from build123d import *

# Parameters (mm, degrees)
BOSS_EXTRUDE1_DEPTH = 2.54
CUT_EXTRUDE1_DEPTH  = 3.54
CUT_EXTRUDE2_DEPTH  = 3.54


with BuildPart() as part:
    # Sketch1 → Boss-Extrude1 (new body)
    with BuildSketch(Plane(origin=(0, 0, 0), x_dir=(1, 0, 0), z_dir=(0, 1, 0))):
        Polygon((-66.675, 25.4), (-69.215, 25.4), (-69.215, -25.4), (-66.675, -25.4), (-66.675, -27.813), (66.675, -27.813), (66.675, -25.4), (69.215, -25.4), (69.215, 25.4), (66.675, 25.4), (66.675, 27.813), (-66.675, 27.813), align=None)
    extrude(amount=BOSS_EXTRUDE1_DEPTH)

    # Sketch2 → Cut-Extrude1 (cut, through all)
    with BuildSketch(Plane(origin=(0, 2.54, 0), x_dir=(1, 0, 0), z_dir=(0, 1, 0))):
        with BuildLine():
            ThreePointArc((-60.96, 16.51), (-64.212038418, 17.857038418), (-62.865, 14.605))
            Line((-62.865, 14.605), (-62.865, 16.51))
            Line((-62.865, 16.51), (-60.96, 16.51))
        make_face()
        with BuildLine():
            Line((-62.865, 16.51), (-62.865, 14.605))
            ThreePointArc((-62.865, 14.605), (-61.517961582, 15.162961582), (-60.96, 16.51))
            Line((-60.96, 16.51), (-62.865, 16.51))
        make_face()
        with BuildLine():
            ThreePointArc((-19.05, 16.51), (-18.492038418, 15.162961582), (-17.145, 14.605))
            Line((-17.145, 14.605), (-17.145, 16.51))
            Line((-17.145, 16.51), (-19.05, 16.51))
        make_face()
        with BuildLine():
            Line((-17.145, 16.51), (-17.145, 14.605))
            ThreePointArc((-17.145, 14.605), (-15.797961582, 15.162961582), (-15.24, 16.51))
            ThreePointArc((-15.24, 16.51), (-17.145, 18.415), (-19.05, 16.51))
            Line((-19.05, 16.51), (-17.145, 16.51))
        make_face()
        with BuildLine():
            ThreePointArc((-17.145, -14.605), (-18.492038418, -15.162961582), (-19.05, -16.51))
            Line((-19.05, -16.51), (-17.145, -16.51))
            Line((-17.145, -16.51), (-17.145, -14.605))
        make_face()
        with BuildLine():
            Line((-17.145, -16.51), (-19.05, -16.51))
            ThreePointArc((-19.05, -16.51), (-17.145, -18.415), (-15.24, -16.51))
            ThreePointArc((-15.24, -16.51), (-15.797961582, -15.162961582), (-17.145, -14.605))
            Line((-17.145, -14.605), (-17.145, -16.51))
        make_face()
        with BuildLine():
            Line((-62.865, -14.605), (-62.865, -16.51))
            Line((-62.865, -16.51), (-60.96, -16.51))
            ThreePointArc((-60.96, -16.51), (-61.517961582, -15.162961582), (-62.865, -14.605))
        make_face()
        with BuildLine():
            Line((-60.96, -16.51), (-62.865, -16.51))
            Line((-62.865, -16.51), (-62.865, -14.605))
            ThreePointArc((-62.865, -14.605), (-64.212038418, -17.857038418), (-60.96, -16.51))
        make_face()
    extrude(amount=-CUT_EXTRUDE1_DEPTH, mode=Mode.SUBTRACT)

    # Sketch3 → Cut-Extrude2 (cut, through all)
    with BuildSketch(Plane(origin=(0, 2.54, 0), x_dir=(1, 0, 0), z_dir=(0, 1, 0))):
        with BuildLine():
            Line((44.1325, 15.8877), (44.1325, 15.8623))
            ThreePointArc((44.1325, 15.8623), (43.671251759, 14.748748241), (42.5577, 14.2875))
            Line((42.5577, 14.2875), (26.6573, 14.2875))
            ThreePointArc((26.6573, 14.2875), (25.543748241, 14.748748241), (25.0825, 15.8623))
            Line((25.0825, 15.8623), (25.0825, 15.8877))
            ThreePointArc((25.0825, 15.8877), (25.543748241, 17.001251759), (26.6573, 17.4625))
            Line((26.6573, 17.4625), (42.5577, 17.4625))
            ThreePointArc((42.5577, 17.4625), (43.671251759, 17.001251759), (44.1325, 15.8877))
        make_face()
        with BuildLine():
            Line((42.5577, -17.4625), (26.6573, -17.4625))
            ThreePointArc((26.6573, -17.4625), (25.543748241, -17.001251759), (25.0825, -15.8877))
            Line((25.0825, -15.8877), (25.0825, -15.8623))
            ThreePointArc((25.0825, -15.8623), (25.543748241, -14.748748241), (26.6573, -14.2875))
            Line((26.6573, -14.2875), (42.5577, -14.2875))
            ThreePointArc((42.5577, -14.2875), (43.671251759, -14.748748241), (44.1325, -15.8623))
            Line((44.1325, -15.8623), (44.1325, -15.8877))
            ThreePointArc((44.1325, -15.8877), (43.671251759, -17.001251759), (42.5577, -17.4625))
        make_face()
    extrude(amount=-CUT_EXTRUDE2_DEPTH, mode=Mode.SUBTRACT)


solid = part.part
Read the model definition and answer for the solid it produces. Units are mm, in the model's axes. A direction names the side the tool comes from. Round coordinates to 2 decimals unless told otherwise and drop trailing zeros. Use a Markdown table: item, result.
(1) Each of these flat-tipped pins is pushed along its axis until it touches: pin 1 Ø1.2 at (y, z) = (1, -26.5) entering from +X (3 decimals); pin 2 Ø1.3 at (x, y) = (68, 1.5) entering from -Z; pin 3 Ø2 at (x, z) = (50.5, -10) entering from -Y. Where does it stop, or does it pass through?
Reported:
| item | result |
|---|---|
| pin 1 | x = 66.675 |
| pin 2 | z = -25.4 |
| pin 3 | y = 0 |
(2) The mould has two halves that part along X. Classify faces 1 (the flat face through (34, 1, 14.288)), 2 (the flat face through (69.215, 1, 0)), 3 (the flat face through (-1, 0, 0)): released by +X, released by -X, zero draft, split by the parting line, or undercut.
Reported:
| item | result |
|---|---|
| face 1 | undercut |
| face 2 | released by +X |
| face 3 | zero draft |
(3) Which of the six approach directions +Z, -Z, +X, -X, +Y, -Y give full straight-line access (tool end or side, diameter ignored) to faces 4 (the flat face through (66.675, 1, -27)), 5 (the flat face through (-68, 1, 25.4)), 6 (the flat face through (68, 1, 25.4)), 7 (the flat face through (35, 1, 17.462))?
Reported:
| item | result |
|---|---|
| face 4 | -Z, +X, +Y, -Y |
| face 5 | +Z, -X, +Y, -Y |
| face 6 | +Z, +X, +Y, -Y |
| face 7 | +Y, -Y |
(4) The part is cut by section A-A (y = 1.35). State how many separate pieces and enclosed holes the cut face has, then the cut area to 3 significant figures.
Reported:
| item | result |
|---|---|
| separate pieces | 1 |
| enclosed holes | 6 |
| area | 7,510 mm2 |
(5) Straight lines are drawn through the part: line 1 along X through (y, z) = (1.4, -16.51) (3 decimals); line 2 along Z through (x, y) = (33, 0.6); line 3 along X through (y, z) = (0.2, 16) (1 decimal). For each, find the intervals that lie inside material, in ascending order. Write a range as [from, to].
Reported:
| item | result |
|---|---|
| line 1 | [-69.215, -64.77], [-60.96, -19.05], [-15.24, 25.211], [44.004, 69.215] |
| line 2 | [-27.81, -17.46], [-14.29, 14.29], [17.46, 27.81] |
| line 3 | [-69.2, -64.7], [-61, -19], [-15.3, 25.1], [44.1, 69.2] |
